Answer from the drawing. Dimensions are ordinates in mm from the lowest x, y and z of the part. A direction names the side the tool comes from. Give positions to 0.01 mm unless a question says otherwise; leave off trailing zeros. Loops run counter-clockwise (first coordinate to the right, second up) from the corner with the lowest first, then second, coordinate; pieces in that order, holes last. Notation, with made-up numbers: (2.25, 34) - (38.25, 34) arc R3 ccw to (38.25, 39) - close; hole circle Ø3 at (43.25, 61.5). An arc over 180 degrees is marked (long way). One line per question, with ' | ' between items. Start each with the question number.
1. Each of these flat-tipped pins is pushed along its axis until it touches: pin 1 (5 mm diameter, centred on y = 28.5, z = 18.5, fed in from -X); pin 2 (1.5 mm diameter, centred on x = 4.5, y = 91, fed in from +Z); pin 3 (1 mm diameter, centred on x = 4.5, z = 17, fed in from -Y). Where does it stop, or does it pass through?
2. Which of the six approach directions +Z, -Z, +X, -X, +Y, -Y give full straight-line access (tool end or side, diameter ignored) to the marked faces 1 and 2?
3. Section C-C (y = 52.5) is taken. Determine the outline of the cut face in (x, z) (3 decimals).
4. Find the intervals of material crossed by line 1 (Z direction, x = 3, y = 94); line 2 (Y direction, x = 5, z = 48); line 3 (Y direction, x = 2.5, z = 16), in increasing order.
5. Section B-B (z = 43.5) is taken. Determine the outline of the cut face in (x, y) (3 decimals).
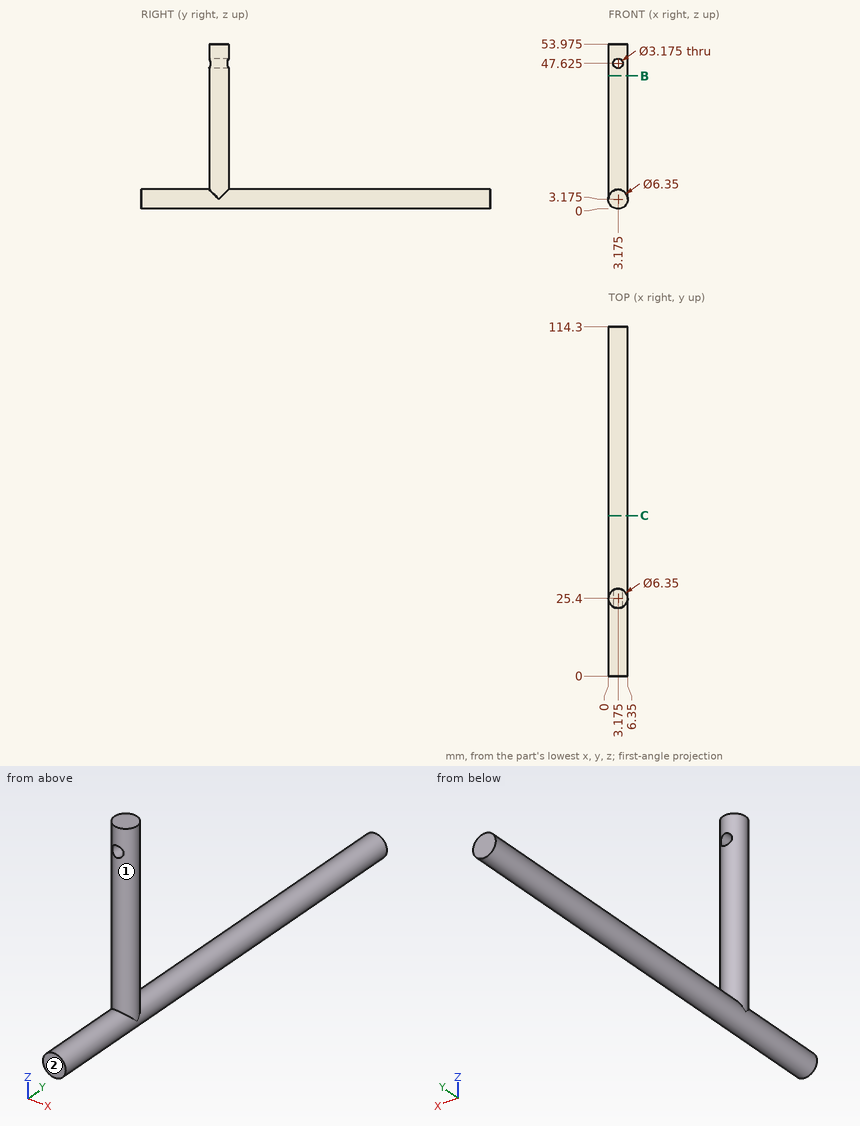
Conclusion:
1) pin 1: x = 0.06 | pin 2: z = 6.3 | pin 3: y = 22.33
2) face 1: +Z | face 2: +Z, -Z, +X, -X, -Y
3) outline: circle Ø6.35 at (3.175, 3.175)
4) line 1: 0 to 6.35 | line 2: 22.8 to 28 | line 3: 22.3 to 28.5
5) outline: circle Ø6.35 at (3.175, 25.4)
